Input: part model. Units: mm. Frame: model coordinates. Face numbers are marked on the shaded views. A direction names the side the tool comes from. Round coordinates to 2 decimals unless told otherwise and drop trailing zeros. Write each loop counter-clockwise with the first axis right and the second up, starting at its lowest first coordinate (ties: lowest second). Pieces come first, ordered by that corner, then holes. Notation, with made-up numbers: (43, 44) -> (99, 44) arc R31 ccw to (99, 79) -> close; hole circle Ø8 at (-23, 33). An arc over 180 degrees is marked (long way). Write item = value, one per line.
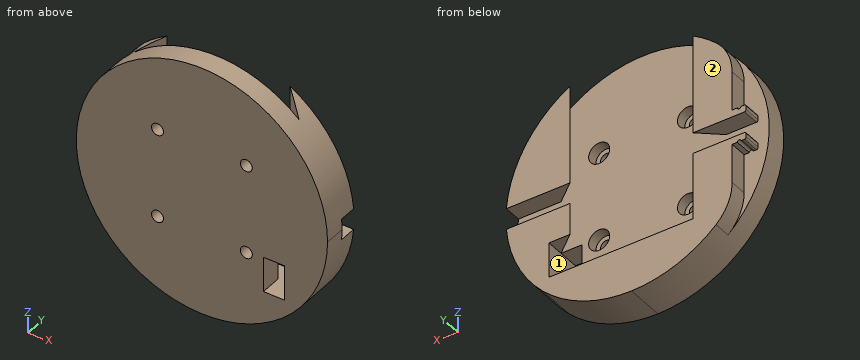
```python
from build123d import *

# Parameters (mm, degrees)
SKETCH1_R                      = 1.7
BOSS_EXTRUDE1_DEPTH            = 11
CUT_EXTRUDE1_START             = -8
SKETCH2_R                      = 3
SKETCH2_R_2                    = 1.7
CUT_EXTRUDE1_DEPTH             = 8
SKETCH3_W                      = 6
SKETCH3_H                      = 10
CUT_EXTRUDE2_DEPTH             = 34
CUT_EXTRUDE3_REACH             = 53.741
SKETCH4_W                      = 35
SKETCH4_H                      = 5
CUT_EXTRUDE3_DIRECTION_2_DEPTH = 44
CUT_EXTRUDE4_DEPTH             = 71.068716272
CUT_EXTRUDE4_DEPTH_BACK        = 71.068716272
CUT_EXTRUDE5_DEPTH             = 5
FILLET3_R                      = 0.5
FILLET4_R                      = 14


with BuildPart() as part:
    # Sketch1 → Boss-Extrude1 (new body)
    # profile 1 of 3: a face of its own
    with BuildSketch(Plane(origin=(0, 0, 0), x_dir=(1, 0, 0), z_dir=(0, 1, 0))):
        with BuildLine():
            Line((35.75, 0), (0, 0))
            Line((0, 0), (0, 35.75))
            ThreePointArc((0, 35.75), (-25.279067427, -25.279067427), (35.75, 0))
        make_face()
        with Locations(Location((-12.639533714, -12.639533714, 0), (0, 0, 270))):
            Circle(SKETCH1_R, mode=Mode.SUBTRACT)
        with Locations(Location((12.639533714, -12.639533714, 0), (0, 0, 270))):
            Circle(SKETCH1_R, mode=Mode.SUBTRACT)
        with Locations(Location((-12.639533714, 12.639533714, 0), (0, 0, 270))):
            Circle(SKETCH1_R, mode=Mode.SUBTRACT)
    # profile 2 of 3: a face of its own
    with BuildSketch(Plane(origin=(0, 0, 0), x_dir=(1, 0, 0), z_dir=(0, 1, 0))):
        with BuildLine():
            Line((0, 35.75), (0, 0))
            Line((0, 0), (11.437452186, 11.437452186))
            ThreePointArc((11.437452186, 11.437452186), (11.437452186, 13.841615242), (13.841615242, 13.841615242))
            Line((13.841615242, 13.841615242), (25.279067427, 25.279067427))
            ThreePointArc((25.279067427, 25.279067427), (13.680932707, 33.028693287), (0, 35.75))
        make_face()
    # profile 3 of 3: a face of its own
    with BuildSketch(Plane(origin=(0, 0, 0), x_dir=(1, 0, 0), z_dir=(0, 1, 0))):
        with BuildLine():
            Line((11.437452186, 11.437452186), (0, 0))
            Line((0, 0), (35.75, 0))
            ThreePointArc((35.75, 0), (33.028693287, 13.680932707), (25.279067427, 25.279067427))
            Line((25.279067427, 25.279067427), (13.841615242, 13.841615242))
            ThreePointArc((13.841615242, 13.841615242), (14.210128919, 13.290095549), (14.339533714, 12.639533714))
            ThreePointArc((14.339533714, 12.639533714), (13.290095549, 11.068938508), (11.437452186, 11.437452186))
        make_face()
    extrude(amount=BOSS_EXTRUDE1_DEPTH)

    # Sketch2 → Cut-Extrude1 (cut)
    # profile 1 of 4: a face of its own
    with BuildSketch(Plane(origin=(0, 11, 0), x_dir=(1, 0, 0), z_dir=(0, 1, 0)).offset(CUT_EXTRUDE1_START)):
        with Locations(Location((-12.639533714, -12.639533714, 0), (0, 0, 270))):
            Circle(SKETCH2_R)
        with Locations(Location((-12.639533714, -12.639533714, 0), (0, 0, 270))):
            Circle(SKETCH2_R_2, mode=Mode.SUBTRACT)
    # profile 2 of 4: a face of its own
    with BuildSketch(Plane(origin=(0, 11, 0), x_dir=(1, 0, 0), z_dir=(0, 1, 0)).offset(CUT_EXTRUDE1_START)):
        with Locations(Location((12.639533714, -12.639533714, 0), (0, 0, 270))):
            Circle(SKETCH2_R)
        with Locations(Location((12.639533714, -12.639533714, 0), (0, 0, 270))):
            Circle(SKETCH2_R_2, mode=Mode.SUBTRACT)
    # profile 3 of 4: a face of its own
    with BuildSketch(Plane(origin=(0, 11, 0), x_dir=(1, 0, 0), z_dir=(0, 1, 0)).offset(CUT_EXTRUDE1_START)):
        with Locations(Location((12.639533714, 12.639533714, 0), (0, 0, 270))):
            Circle(SKETCH2_R)
        with Locations(Location((12.639533714, 12.639533714, 0), (0, 0, 270))):
            Circle(SKETCH2_R_2, mode=Mode.SUBTRACT)
    # profile 4 of 4: a face of its own
    with BuildSketch(Plane(origin=(0, 11, 0), x_dir=(1, 0, 0), z_dir=(0, 1, 0)).offset(CUT_EXTRUDE1_START)):
        with Locations(Location((-12.639533714, 12.639533714, 0), (0, 0, 270))):
            Circle(SKETCH2_R)
        with Locations(Location((-12.639533714, 12.639533714, 0), (0, 0, 270))):
            Circle(SKETCH2_R_2, mode=Mode.SUBTRACT)
    extrude(amount=CUT_EXTRUDE1_DEPTH, mode=Mode.SUBTRACT)

    # Sketch3 → Cut-Extrude2 (cut)
    with BuildSketch(Plane(origin=(0, 11, 0), x_dir=(1, 0, 0), z_dir=(0, 1, 0))):
        with Locations((20.5, 17)):
            Rectangle(SKETCH3_W, SKETCH3_H)
    extrude(amount=-CUT_EXTRUDE2_DEPTH, mode=Mode.SUBTRACT)

    # Cut-Extrude3: up to this face of the body (flat: up to its plane)
    cut_extrude3_end = Plane(part.part.faces().sort_by_distance((20.5, 5.5, -22))[0])
    # Sketch4 → Cut-Extrude3 (cut, up to the picked face)
    with BuildSketch(Plane.XY, mode=Mode.PRIVATE) as cut_extrude3_sk1:
        with Locations((0, 8.5)):
            Rectangle(SKETCH4_W, SKETCH4_H)
    cut_extrude3_tool1 = split(extrude(cut_extrude3_sk1.sketch, amount=-CUT_EXTRUDE3_REACH, mode=Mode.PRIVATE), bisect_by=cut_extrude3_end, keep=Keep.BOTH, mode=Mode.PRIVATE)
    # Sketch4 → Cut-Extrude3 (cut, up to the picked face)
    with BuildSketch(Plane.XY, mode=Mode.PRIVATE) as cut_extrude3_sk2:
        Polygon((-17.5, 6), (-17.5, 11), (-23.5, 6), align=None)
    cut_extrude3_tool2 = split(extrude(cut_extrude3_sk2.sketch, amount=-CUT_EXTRUDE3_REACH, mode=Mode.PRIVATE), bisect_by=cut_extrude3_end, keep=Keep.BOTH, mode=Mode.PRIVATE)
    # Sketch4 → Cut-Extrude3 (cut, up to the picked face)
    with BuildSketch(Plane.XY, mode=Mode.PRIVATE) as cut_extrude3_sk3:
        Polygon((23.5, 6), (17.5, 6), (17.5, 11), align=None)
    cut_extrude3_tool3 = split(extrude(cut_extrude3_sk3.sketch, amount=-CUT_EXTRUDE3_REACH, mode=Mode.PRIVATE), bisect_by=cut_extrude3_end, keep=Keep.BOTH, mode=Mode.PRIVATE)
    add(cut_extrude3_tool1.solids().sort_by(Axis((0, 8.5, 0), (0, 0, -1)))[0], mode=Mode.SUBTRACT)
    add(cut_extrude3_tool2.solids().sort_by(Axis((-19.5, 7.666667, 0), (0, 0, -1)))[0], mode=Mode.SUBTRACT)
    add(cut_extrude3_tool3.solids().sort_by(Axis((19.5, 7.666667, 0), (0, 0, -1)))[0], mode=Mode.SUBTRACT)

    # Sketch4 → Cut-Extrude3 direction 2 (cut)
    with BuildSketch(Plane.XY):
        with Locations((0, 8.5)):
            Rectangle(SKETCH4_W, SKETCH4_H)
        Polygon((-17.5, 6), (-17.5, 11), (-23.5, 6), align=None)
        Polygon((23.5, 6), (17.5, 6), (17.5, 11), align=None)
    extrude(amount=CUT_EXTRUDE3_DIRECTION_2_DEPTH, mode=Mode.SUBTRACT)

    # Sketch5 → Cut-Extrude4 (cut, two sides: drawn at the far end of the back side and taken through both)
    with BuildSketch(Plane.ZY.offset(-23.5).offset(-CUT_EXTRUDE4_DEPTH_BACK)):
        Polygon((-3, 11), (-3, 6), (0, 6), (3, 6), (3, 11), align=None)
    extrude(amount=CUT_EXTRUDE4_DEPTH + CUT_EXTRUDE4_DEPTH_BACK, mode=Mode.SUBTRACT)

    # Sketch6 → Cut-Extrude5 (cut)
    with BuildSketch(Plane(origin=(0, 11, 0), x_dir=(1, 0, 0), z_dir=(0, 1, 0))):
        Polygon((-35.623903492, 21.174718123), (-35.623903492, 3), (-32.623903492, 3), (-32.623903492, 5), (-32.623903492, 21.174718123), align=None)
        with BuildLine():
            Line((-35.623903492, 31.403345095), (-35.623903492, 21.174718123))
            Line((-35.623903492, 21.174718123), (-32.623903492, 21.174718123))
            Line((-32.623903492, 21.174718123), (-32.623903492, 5))
            Line((-32.623903492, 5), (-31.123903492, 5))
            ThreePointArc((-31.123903492, 5), (-30.623903492, 5.5), (-30.123903492, 5))
            Line((-30.123903492, 5), (-28.623903492, 5))
            Line((-28.623903492, 5), (-28.623903492, 18.959009746))
            Line((-28.623903492, 18.959009746), (-28.623903492, 31.403345095))
            Line((-28.623903492, 31.403345095), (-35.623903492, 31.403345095))
        make_face()
        with BuildLine():
            ThreePointArc((-30.123903492, 5), (-30.623903492, 5.5), (-31.123903492, 5))
            Line((-31.123903492, 5), (-30.123903492, 5))
        make_face()
        with BuildLine():
            Line((-30.123903492, 5), (-31.123903492, 5))
            ThreePointArc((-31.123903492, 5), (-30.623903492, 4.5), (-30.123903492, 5))
        make_face()
        with BuildLine():
            Line((-32.623903492, -5), (-32.623903492, -21.174718123))
            Line((-32.623903492, -21.174718123), (-35.623903492, -21.174718123))
            Line((-35.623903492, -21.174718123), (-35.623903492, -31.403345095))
            Line((-35.623903492, -31.403345095), (-28.623903492, -31.403345095))
            Line((-28.623903492, -31.403345095), (-28.623903492, -5))
            Line((-28.623903492, -5), (-30.123903492, -5))
            ThreePointArc((-30.123903492, -5), (-30.623903492, -5.5), (-31.123903492, -5))
            Line((-31.123903492, -5), (-32.623903492, -5))
        make_face()
        Polygon((-35.623903492, -21.174718123), (-32.623903492, -21.174718123), (-32.623903492, -5), (-32.623903492, -3), (-35.623903492, -3), align=None)
        with BuildLine():
            ThreePointArc((-30.123903492, -5), (-30.623903492, -4.5), (-31.123903492, -5))
            Line((-31.123903492, -5), (-30.123903492, -5))
        make_face()
        with BuildLine():
            Line((-30.123903492, -5), (-31.123903492, -5))
            ThreePointArc((-31.123903492, -5), (-30.623903492, -5.5), (-30.123903492, -5))
        make_face()
    extrude(amount=-CUT_EXTRUDE5_DEPTH, mode=Mode.SUBTRACT)

    # Fillet3
    fillet3_edges = [part.edges().sort_by_distance(p)[0] for p in [
        (-31.123903492, 8.5, -5),
        (-32.623903492, 8.5, -5),
        (-32.623903492, 8.5, -3),
        (-31.123903492, 8.5, 5),
        (-32.623903492, 8.5, 5),
        (-32.623903492, 8.5, 3),
    ]]
    fillet(fillet3_edges, radius=FILLET3_R)

    # Fillet4
    fillet4_edges = [part.edges().sort_by_distance(p)[0] for p in [
        (-28.623903492, 8.5, -21.418091626),
        (-28.623903492, 8.5, 21.418091626),
    ]]
    fillet(fillet4_edges, radius=FILLET4_R)


solid = part.part
```
1) First-contact query: P1, Ø5, axis at y = 8.5, z = -25, coming from the +X side; P2, Ø1.5, axis at y = 9.5, z = 18.5, coming from the +X side; P3, Ø5.5, axis at y = 9.5, z = 10.5, coming from the -X side; P4, Ø3.5, axis at x = -12.64, z = -12.64, coming from the -Y side. Flat tips, straight axial feed; report the tip coordinate or a pass-through.
Solutions:
P1 = 27.78
P2 = 31.03
P3 = -28.62
P4 = 0
2) Cut plane A-A (x = -19.5). Return the cut outline in (y, z), and give its area (3 significant figures).
Solutions:
outline = (0, -29.96) -> (11, -29.96) -> (11, -3) -> (9.33, -3) -> (9.33, -22) -> (6, -22) -> (6, 29.96) -> (0, 29.96) -> close; (9.33, 3) -> (11, 3) -> (11, 29.96) -> (9.33, 29.96) -> close
area = 476 mm^2
3) Cut plane D-D (z = 2). Return the cut outline in (x, y).
Solutions:
outline = (-35.69, 0) -> (35.69, 0) -> (35.69, 6) -> (-35.69, 6) -> close
4) Line query: L1, parallel to Y at x = 7.5, z = 2; L2, parallel to Z at x = -29.5, y = 10.5; L3, parallel to X at y = 2.5, z = -13. Output: solid intervals per line, ascending. Write a range as from..to.
Solutions:
L1 = 0..6
L2 = -5..-3, 3..5
L3 = -33.3..-14.3, -10.98..10.98, 14.3..17.5, 23.5..33.3
5) Cut plane C-C (x = 28). Return the cut outline in (y, z).
Solutions:
outline = (0, -22.23) -> (11, -22.23) -> (11, -3) -> (6, -3) -> (6, 3) -> (11, 3) -> (11, 22.23) -> (0, 22.23) -> close
6) Cut plane B-B (x = 20). Return the cut outline in (y, z).
Solutions:
outline = (0, -29.63) -> (11, -29.63) -> (11, -22) -> (0, -22) -> close; (0, -12) -> (6, -12) -> (6, 29.63) -> (0, 29.63) -> close; (8.92, -12) -> (11, -12) -> (11, -3) -> (8.92, -3) -> close; (8.92, 3) -> (11, 3) -> (11, 29.63) -> (8.92, 29.63) -> close
7) Access query for the marked faces 1 and 2. Directions: +Z, -Z, +X, -X, +Y, -Y. A direction counts if a zero-diameter tool reaches every point of the face in a straight line with its end or side. Return the directions, or none.
Solutions:
face_1 = +Y, -Y
face_2 = +Z, -Z, +X, -X, +Y
